Here's the drawing with two shaded views (mm, measured from the low corner). I have some questions. Round coordinates to 2 decimals unless told otherwise and drop trailing zeros. Loops run counter-clockwise (first coordinate to the right, second up) from the corner with the lowest first, then second, coordinate; pieces in that order, holes last. Notation, with made-up numbers: (-29, 36) -> (26, 36) arc R18 cw to (26, 62) -> close; hole circle Ø6 at (41.25, 89.25). An arc over 180 degrees is marked (long way). Write each question's results on one line, items separated by ' | '.
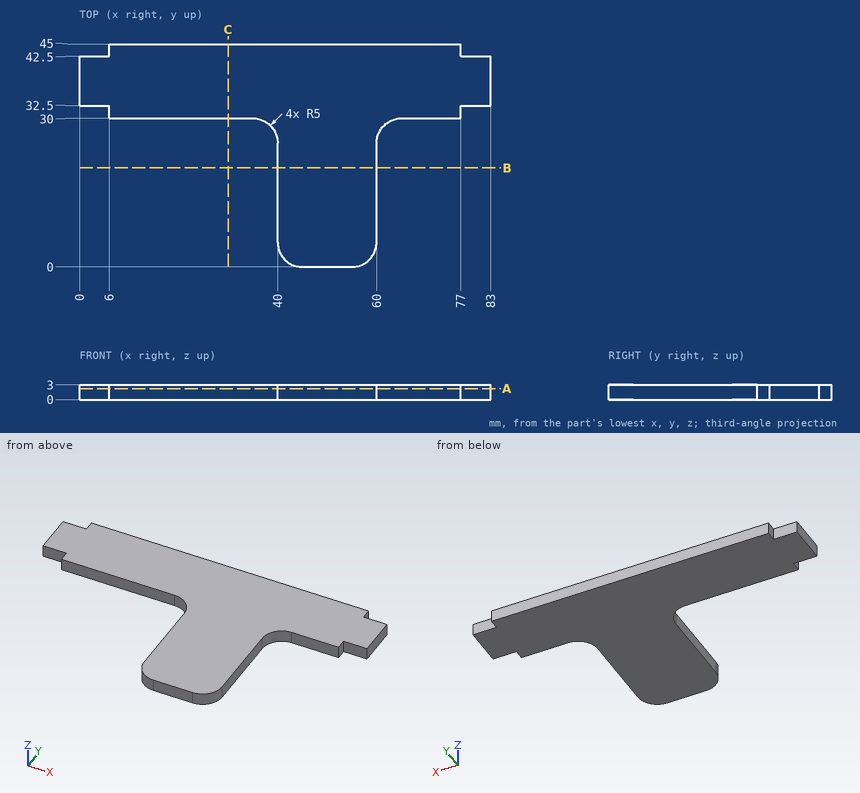
1. If we section it at A-A (z = 2.25): List the corners of the cut face in (x, y) for me.
Final values:
outline: (0, 32.5) -> (6, 32.5) -> (6, 30) -> (35, 30) arc R5 cw to (40, 25) -> (40, 5) arc R5 ccw to (45, 0) -> (55, 0) arc R5 ccw to (60, 5) -> (60, 25) arc R5 cw to (65, 30) -> (77, 30) -> (77, 32.5) -> (83, 32.5) -> (83, 42.5) -> (77, 42.5) -> (77, 45) -> (6, 45) -> (6, 42.5) -> (0, 42.5) -> close
2. Please list where these lines run through material, in increasing order: line 1 (X direction, y = 32, z = 1.7); line 2 (X direction, y = 19.5, z = 2.6); line 3 (Y direction, x = 5, z = 2.6). Write a range as from..to.
Final values:
line 1: 6..77 | line 2: 40..60 | line 3: 32.5..42.5
3. If we section it at C-C (x = 30): List the corners of the cut face in (y, z) for me, then the cut area to 3 significant figures.
Final values:
outline: (30, 0) -> (45, 0) -> (45, 3) -> (30, 3) -> close | area: 45.0 mm2
4. If we section it at B-B (y = 20): List the corners of the cut face in (x, z) for me, then the cut area to 3 significant figures.
Final values:
outline: (40, 0) -> (60, 0) -> (60, 3) -> (40, 3) -> close | area: 60.0 mm2
5. Will these pins go through, and if not, where does the flat tip stop? pin 1 (0.9 mm diameter, centred on x = 20, z = 1, fed in from -Y); pin 2 (1.5 mm diameter, centred on x = 79.5, z = 1, fed in from -Y); pin 3 (0.8 mm diameter, centred on y = 31.5, z = 1, fed in from +X).
Final values:
pin 1: y = 30 | pin 2: y = 32.5 | pin 3: x = 77
